Answer from the drawing. Dimensions are ordinates in mm from the lowest x, y and z of the part. A direction names the side the tool comes from. Coordinates: 2 decimals unless noted, no trailing zeros. Write each loop counter-clockwise with the first axis right and the second up, starting at its lowest first coordinate (ties: lowest second). Pieces come first, ordered by that corner, then holes.
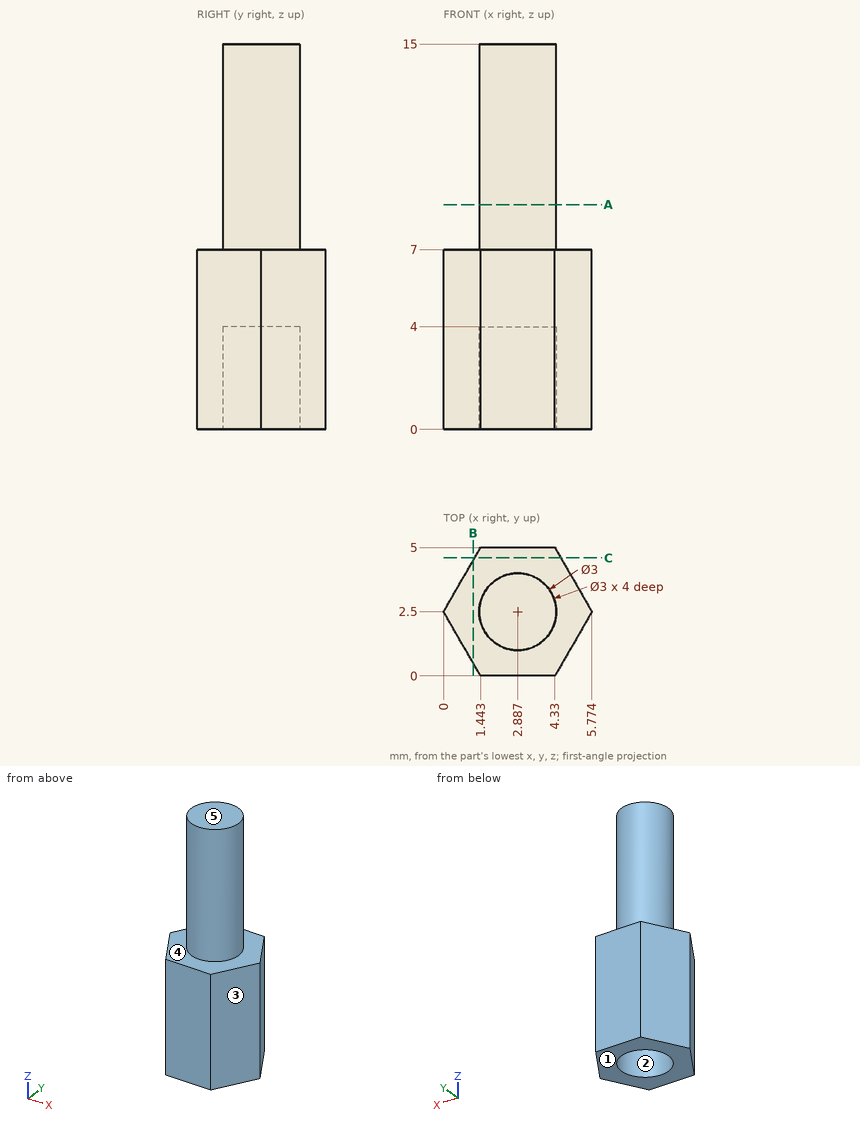
(1) For a pull along X with two mould halves and no side action, classify the marked faces 1, 2 and 3 as pulls with the +X half, pulls with the -X half, needs draft (parallel to the pull), parting line crosses it, or undercut.
(2) This flat-tipped pin is pushed along its axis until it touches: pin 1 (3 mm diameter, centred on y = 3, z = 13, fed in from +X). Where does it stop, or does it pass through?
(3) Which of the six approach directions +Z, -Z, +X, -X, +Y, -Y give full straight-line access (tool end or side, diameter ignored) to the marked faces 4 and 5?
(4) Section B-B, the plane x = 1.15 is taken. Write down the section's boundary in (y, z).
(5) Section C-C, the plane y = 4.6 is taken. Write down the section's boundary in (x, z).
(6) Find the intervals of material crossed by probe 1 along Z at (x, y) = (3.9, 4.7); probe 2 along Z at (x, y) = (2.4, 1.8); probe 3 along X at (y, z) = (1, 6.25) (1 decimal), in increasing order.
(7) Section A-A, the plane z = 8.75 is taken. Write down the section's boundary in (x, y).
Solution:
1. face 1: needs draft
1. face 2: undercut
1. face 3: pulls with the +X half
2. pin 1: stops at x = 4.39
3. face 4: +Z
3. face 5: +Z, +X, -X, +Y, -Y
4. outline: (0.51, 0) - (4.49, 0) - (4.49, 7) - (0.51, 7) - close
5. outline: (1.21, 0) - (4.56, 0) - (4.56, 7) - (1.21, 7) - close
6. probe 1: z = 0 to 7
6. probe 2: z = 4 to 15
6. probe 3: x = 0.9 to 4.9
7. outline: circle Ø3 at (2.89, 2.5)
